from build123d import *

# Parameters (mm, degrees)
F1_W     = 76.2
F1_H     = 38.1
F1_R     = 12.7
F2_DEPTH = 5.08
F3_R     = 12.7
F4_DEPTH = 25.4


# Not quite as in the source:
# - a variable given as a bare number and used for a length is read in inches; the dataset says mm whatever the document's units were


with BuildPart() as f2:
    # F1 (on Top) → F2 (new body)
    with BuildSketch(Plane.XY):
        Rectangle(F1_W, F1_H)
        Circle(F1_R, mode=Mode.SUBTRACT)
    extrude(amount=F2_DEPTH)

    # F3
    f3_edges = [f2.edges().sort_by_distance(p)[0] for p in [
        (38.1, -19.05, 2.54),
        (38.1, 19.05, 2.54),
        (-38.1, -19.05, 2.54),
        (-38.1, 19.05, 2.54),
    ]]
    fillet(f3_edges, radius=F3_R)

    # F1 (on Top) → F4 (join)
    with BuildSketch(Plane.XY):
        Rectangle(F1_W, F1_H)
        Circle(F1_R, mode=Mode.SUBTRACT)
    extrude(amount=-F4_DEPTH)


solid = f2.part
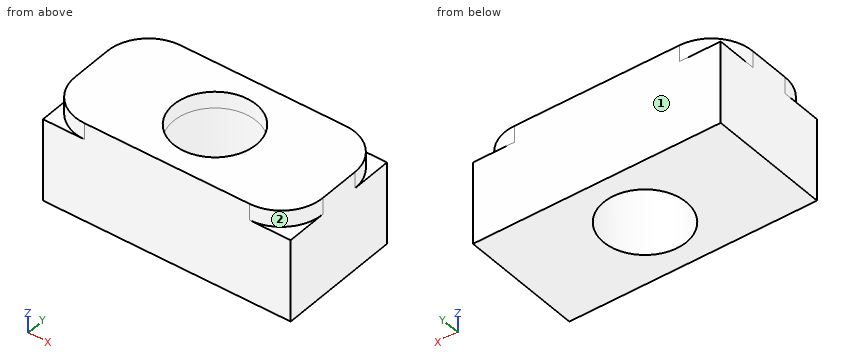
Verification items for the finished model (mm, model axes). Face numbers are marked on the shaded views. A direction names the side the tool comes from. Coordinates: 2 decimals unless noted, no trailing zeros. Order: outer loops, then holes, each group sorted by start corner. A loop starts at its lowest first (then second) coordinate and runs counter-clockwise, first axis right, second up. Notation, with made-up numbers: (72.25, 20) -> (101.25, 20) arc R37 cw to (101.25, 58) -> close; hole circle Ø1 at (-7.75, -29.75). An arc over 180 degrees is marked (long way). Put each result on its own line as item: value. Start each with the question number.
1. Cross-section at B-B, the plane y = 0. Record the boundary of the cut face in (x, z).
2. Cross-section at D-D, the plane y = 9. Record the boundary of the cut face in (x, z).
3. Cross-section at C-C, the plane z = -22.5. Record the boundary of the cut face in (x, y).
4. Access from +Z, -Z, +X, -X, +Y, -Y to the whole of each face (thin tool, end or side, straight path). Record for the marked faces 1 and 2.
5. Material ranges on L1, parallel to X at y = 0.5, z = -3; L2, parallel to Y at x = 0, z = -13.25, recorded low to high. Write a range as [from, to].
6. Cross-section at A-A, the plane x = 0. Record the boundary of the cut face in (y, z).
Computed:
1. outline: (-38.1, -25.4) -> (-12.7, -25.4) -> (-12.7, 5.08) -> (-38.1, 5.08) -> close; (12.7, -25.4) -> (38.1, -25.4) -> (38.1, 5.08) -> (12.7, 5.08) -> close
2. outline: (-38.1, -25.4) -> (-8.96, -25.4) -> (-8.96, 5.08) -> (-37.82, 5.08) -> (-37.82, 0) -> (-38.1, 0) -> close; (8.96, -25.4) -> (38.1, -25.4) -> (38.1, 0) -> (37.82, 0) -> (37.82, 5.08) -> (8.96, 5.08) -> close
3. outline: (-38.1, -19.05) -> (38.1, -19.05) -> (38.1, 19.05) -> (-38.1, 19.05) -> close; hole circle Ø25.4 at (0, 0)
4. face 1: +Z, -Z, +X, -X, +Y
4. face 2: +Z, +X, -Y
5. L1: [-38.1, -12.69], [12.69, 38.1]
5. L2: [-19.05, -12.7], [12.7, 19.05]
6. outline: (-19.05, -25.4) -> (-12.7, -25.4) -> (-12.7, 5.08) -> (-19.05, 5.08) -> close; (12.7, -25.4) -> (19.05, -25.4) -> (19.05, 5.08) -> (12.7, 5.08) -> close
